Could you check a few things on this model? Use its own coordinates, in mm. Face numbers are marked on the shaded views. A direction names the side the tool comes from. Round coordinates to 2 decimals unless told otherwise and drop trailing zeros. Loops run counter-clockwise (first coordinate to the right, second up) from the corner with the lowest first, then second, coordinate; pieces in that order, holes last. Notation, with made-up numbers: (49.5, -27.75) -> (97.5, -27.75) arc R35 ccw to (97.5, 7.25) -> close; hole circle Ø7 at (21.5, 78.25). An arc over 180 degrees is marked (long way). Put each result on its own line as item: value. Start each with the question number.
1. Which directions (+Z, -Z, +X, -X, +Y, -Y) give clear straight access to the entire face, cutting with the end or side of a thin tool? Please do the marked faces 5, 6 and 7.
2. Imagine slicing it at A-A, the plane x = 47.5. Please give me the cut outline in (y, z), and give its area (3 significant figures).
3. I'm going to push flat-ended pins straight in: P1, Ø12.5, axis at y = 17.5, z = 16, coming from the -X side; P2, Ø5, axis at x = 5.715, z = 27.94, coming from the +Y side; P3, Ø5, axis at x = 17, y = 14.5, coming from the +Z side. Where does each tip first touch, or does it pass through?
4. Imagine slicing it at B-B, the plane z = 24. Please give me the cut outline in (x, y), and give its area (3 significant figures).
5. I need wall thicknesses on line 1 (X direction, y = -4, z = 10); line 2 (X direction, y = 11, z = 13); line 3 (X direction, y = -4, z = 27). Which ranges of each line are inside material? Lowest first, please. Write a range as [from, to].
6. Imagine slicing it at D-D, the plane z = 27.94. Please give me the cut outline in (x, y), and give its area (3 significant figures).
7. Imagine slicing it at C-C, the plane y = -2. Please give me the cut outline in (x, z) (1 decimal), and give its area (3 significant figures).
8. If we mould it in two halves opening along Z, with no side actions, what happens to the marked faces 1, 2, 3 and 4? For each: pulls with the +Z half, pulls with the -Z half, needs draft (parallel to the pull), parting line crosses it, or undercut.
```python
from build123d import *

# Parameters (mm, degrees)
F0_R     = 1.5875
F1_DEPTH = 6.35
F3_DEPTH = 3.175
F5_DEPTH = 3.175


with BuildPart() as f1:
    # F0 (on Front) → F1 (new body)
    with BuildSketch(Plane.XZ):
        Polygon((0, 19.05), (0, 0), (27.627938, 0), (27.627938, 7.14375), (16.66875, 7.14375), (16.66875, 19.05), align=None)
        with Locations((5.715, 10.16)):
            Circle(F0_R, mode=Mode.SUBTRACT)
        Polygon((27.627938, 7.14375), (27.627938, 0), (63.5, 0), (63.5, 22.522444), (46.83125, 22.522444), (46.83125, 7.14375), align=None)
        with Locations((57.785, 10.16)):
            Circle(F0_R, mode=Mode.SUBTRACT)
        Polygon((0, 38.1), (0, 19.05), (16.66875, 19.05), (16.66875, 30.95625), (31.060793, 30.95625), (31.060793, 38.1), align=None)
        with Locations((5.715, 27.94)):
            Circle(F0_R, mode=Mode.SUBTRACT)
        Polygon((46.83125, 22.522444), (63.5, 22.522444), (63.5, 38.1), (31.060793, 38.1), (31.060793, 30.95625), (46.83125, 30.95625), align=None)
        with Locations((57.785, 27.94)):
            Circle(F0_R, mode=Mode.SUBTRACT)
    extrude(amount=F1_DEPTH)

    # F2 (on face) → F3 (join)
    with BuildSketch(Plane.YZ.offset(16.66875)):
        Polygon((25.556482, 19.414963), (0.168447, 31.315604), (0, 31.394564), (0, 30.95625), (0, 7.14375), (0, 6.705436), (0.168447, 6.784396), (25.566136, 18.689563), (26.335069, 19.05), align=None)
    extrude(amount=-F3_DEPTH)

    # F4 (on face) → F5 (join)
    with BuildSketch(Plane(origin=(46.83125, 0, 0), x_dir=(0, -1, 0), z_dir=(-1, 0, 0))):
        Polygon((-0.168447, 31.315604), (-26.335069, 19.05), (-0.168447, 6.784396), (0, 6.705436), (0, 31.394564), align=None)
    extrude(amount=-F5_DEPTH)


solid = f1.part
```
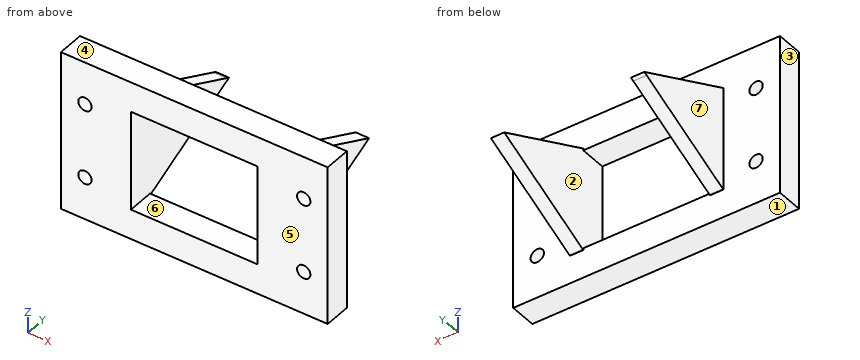
Entries:
1. face 5: +Z, -Z, +X, -X, -Y
1. face 6: +Y, -Y
1. face 7: +Z, -Z, -X, +Y
2. outline: (-6.35, 0) -> (0, 0) -> (0, 6.71) -> (0.17, 6.78) -> (26.34, 19.05) -> (0.17, 31.32) -> (0, 31.39) -> (0, 38.1) -> (-6.35, 38.1) -> close
2. area: 567 mm^2
3. P1: x = 13.49
3. P2: y = 0
3. P3: z = 25.76
4. outline: (0, -6.35) -> (16.67, -6.35) -> (16.67, 15.78) -> (13.49, 15.78) -> (13.49, 0) -> (0, 0) -> close; (46.83, -6.35) -> (63.5, -6.35) -> (63.5, 0) -> (50.01, 0) -> (50.01, 15.78) -> (46.83, 15.78) -> close
4. area: 312 mm^2
5. line 1: [0, 4.14], [7.29, 16.67], [46.83, 56.21], [59.36, 63.5]
5. line 2: [13.49, 16.67], [46.83, 50.01]
5. line 3: [0, 4.44], [6.99, 16.67], [46.83, 56.51], [59.06, 63.5]
6. outline: (0, -6.35) -> (4.13, -6.35) -> (4.13, 0) -> (0, 0) -> close; (7.3, -6.35) -> (16.67, -6.35) -> (16.67, 7.37) -> (13.49, 7.37) -> (13.49, 0) -> (7.3, 0) -> close; (46.83, -6.35) -> (56.2, -6.35) -> (56.2, 0) -> (50.01, 0) -> (50.01, 7.37) -> (46.83, 7.37) -> close; (59.37, -6.35) -> (63.5, -6.35) -> (63.5, 0) -> (59.37, 0) -> close
6. area: 218 mm^2
7. outline: (0, 0) -> (63.5, 0) -> (63.5, 38.1) -> (0, 38.1) -> close; hole circle Ø3.2 at (5.7, 10.2); hole circle Ø3.2 at (5.7, 27.9); hole (16.7, 7.1) -> (46.8, 7.1) -> (46.8, 31) -> (16.7, 31) -> close; hole circle Ø3.2 at (57.8, 10.2); hole circle Ø3.2 at (57.8, 27.9)
7. area: 1,670 mm^2
8. face 1: pulls with the -Z half
8. face 2: undercut
8. face 3: needs draft
8. face 4: pulls with the +Z half
